Autodesk Inventor part; units mm, degrees
ref_plane "Arbeitsebene1" through (0, 0, 17) normal (0, 0, 1) x (1, 0, 0)
ref_plane "Arbeitsebene2" through (32.875, 16, 0) normal (0, 1, 0) x (-1, 0, 0)
ref_plane "YZ Plane" through (0, 0, 0) normal (1, 0, 0) x (0, 1, 0)
sketch "Skizze1" plane through (0, 0, 0) normal (0, 0, 1) x (1, 0, 0)
  line L0 (-95.375, 0) -> (-95.375, -16)
  line L1 (-95.375, -16) -> (-34.625, -16)
  line L2 (-34.625, -16) -> (-34.625, -22)
  line L3 (-34.625, -22) -> (-29.625, -22)
  line L4 (-29.625, -22) -> (-29.625, -16)
  line L5 (-29.625, -16) -> (95.375, -16)
  line L6 (95.375, -16) -> (95.375, 0)
  line L7 (0, -26.4) -> (0, 4.4)
  line L8 (-95.375, 0) -> (95.375, 0)
  point P0 (0, 0)
  dimension "d0" = 190.75
  dimension "d1" = 60.75
  dimension "d2" = 5
  dimension "d3" = 44
  dimension "d4" = 32
revolve "Umdrehung1" add sketch "Skizze1" angle 360 about axis through (-95.375, 0, 0) along (1, 0, 0)
sketch "Skizze2" plane through (95.375, 0, 0) normal (1, 0, 0) x (0, 0, -1)
  point P0 (0, 0)
  point P1 (0, 0)
hole "Bohrung1" at (95.375, 0, 0) direction (-1, 0, 0) diameter 15 depth 15 tip angle 118
ref_plane "Arbeitsebene1" through (0, 0, 17) normal (0, 0, 1) x (1, 0, 0)
sketch "Skizze3" plane through (0, 0, 17) normal (0, 0, 1) x (1, 0, 0)
  line L0 (95.375, 16) -> (95.375, -16)
  line L1 (-19.1, 0) -> (114.6, 0)
  point P0 (0, 0)
  point P1 (89.375, 0)
  dimension "d14" = 6
hole "Bohrung2" at (89.375, 0, 17) direction (0, 0, -1) diameter 3.3 depth 15 tip angle 118
thread "Gewinde1"
ref_plane "Arbeitsebene2" through (32.875, 16, 0) normal (0, 1, 0) x (-1, 0, 0)
sketch "Skizze4" plane through (32.875, 16, 0) normal (0, 1, 0) x (-1, 0, 0)
  line L0 (-51.236, 14.9255) -> (-64.8567, 14.9255)
  line L1 (-64.8567, 14.9255) -> (-64.8567, 17.1103)
  line L2 (-64.8567, 17.1103) -> (-51.236, 17.1103)
  line L3 (-51.236, 17.1103) -> (-51.236, 14.9255)
  point P0 (32.875, 0)
extrude "Extrusion1" cut sketch "Skizze4" against normal through all
sketch "Skizze5" plane through (-95.375, 0, 0) normal (-1, 0, 0) x (0, 0, 1)
  line L0 (-30.8, 0) -> (30.8, 0)
  line L1 (0, -30.8) -> (0, 30.8)
  point P0 (9, 0)
  point P1 (-9, 0)
  dimension "d26" = 18
hole "Bohrung3" at (-95.375, 0, 9) at (-95.375, 0, -9) direction (1, 0, 0) diameter 5 depth 16 tip angle 118
thread "Gewinde2"
thread "Gewinde4"
properties part number "KON_Nietmaschine_Dorn" material "Stahl"
Could you check a few things on this model? Use its own coordinates, in mm. A direction names the side the tool comes from. Round coordinates to 2 decimals unless told otherwise and drop trailing zeros. Write each loop counter-clockwise with the first axis right and the second up, starting at its lowest first coordinate (ties: lowest second). Pieces come first, ordered by that corner, then holes. Notation, with made-up numbers: (19.5, -25.75) -> (47.5, -25.75) arc R22 cw to (47.5, -15.75) -> close; hole circle Ø2 at (66.25, 23.25). An arc over 180 degrees is marked (long way). Use a Markdown table: item, result.
1. Which directions (+Z, -Z, +X, -X, +Y, -Y) give clear straight access to the entire face, cutting with the end or side of a thin tool? Please do faces 1 (the face through (-29.625, -1.5, 16.2)), 2 (the face through (-64.57, 3.47, 15.62)), 3 (the face through (91, 1, 14.926)).
Answer key:
| item | result |
|---|---|
| face 1 | +X |
| face 2 | -X |
| face 3 | +Z, +X, +Y, -Y |
2. Please list where these lines run through material, in increasing order: probe 1 along Z at (x, y) = (-84, 0); probe 2 along Z at (x, y) = (91.75, 0); probe 3 along X at (y, z) = (11.5, 13.5) (3 decimals).
Answer key:
| item | result |
|---|---|
| probe 1 | z = -16 to -11.5, -6.5 to 6.5, 11.5 to 16 |
| probe 2 | z = -16 to -7.5, 7.5 to 14.93 |
| probe 3 | x = -34.625 to -29.625 |
3. For pin 1 Ø3 at (y, z) = (0, 9) entering from -X; pin 2 Ø5 at (x, z) = (13.5, 5) entering from +Y; pin 3 Ø8 at (x, y) = (26.5, 9.5) entering from -Z (3 decimals), each with a flat end and sliding along its axis, tell me the tip position at first contact or that it passes through.
Answer key:
| item | result |
|---|---|
| pin 1 | stops at x = -78.77 |
| pin 2 | stops at y = 15.8 |
| pin 3 | stops at z = -15.025 |
4. If we section it at A-A (y = 11.5): List the corners of the cut face in (x, z) for me (3 decimals), then the cut area to 3 significant figures.
Answer key:
| item | result |
|---|---|
| outline | (-95.375, -11.124) -> (-34.625, -11.124) -> (-34.625, -18.755) -> (-29.625, -18.755) -> (-29.625, -11.124) -> (95.375, -11.124) -> (95.375, 11.124) -> (-29.625, 11.124) -> (-29.625, 18.755) -> (-34.625, 18.755) -> (-34.625, 11.124) -> (-95.375, 11.124) -> close |
| area | 4,320 mm^2 |
5. If we section it at B-B (x = -5): List the corners of the cut face in (y, z) for me.
Answer key:
| item | result |
|---|---|
| outline | circle Ø32 at (0, 0) |
6. We'd pull the mould along Y, two halves only. Please class faces 4 (the face through (95.375, 0, -8)), 5 (the face through (-32.09, 4.769, 21.477)), 6 (the face through (90.986, 0.358, 11.067)): +Y half, -Y half, draft (parallel to the pull), parting line (faces both ways), or undercut.
Answer key:
| item | result |
|---|---|
| face 4 | draft |
| face 5 | parting line |
| face 6 | undercut |
